Here's the drawing with two shaded views (mm, measured from the low corner). I have some questions. A direction names the side the tool comes from. Round coordinates to 2 decimals unless told otherwise and drop trailing zeros. Loops run counter-clockwise (first coordinate to the right, second up) from the corner with the lowest first, then second, coordinate; pieces in that order, holes last.
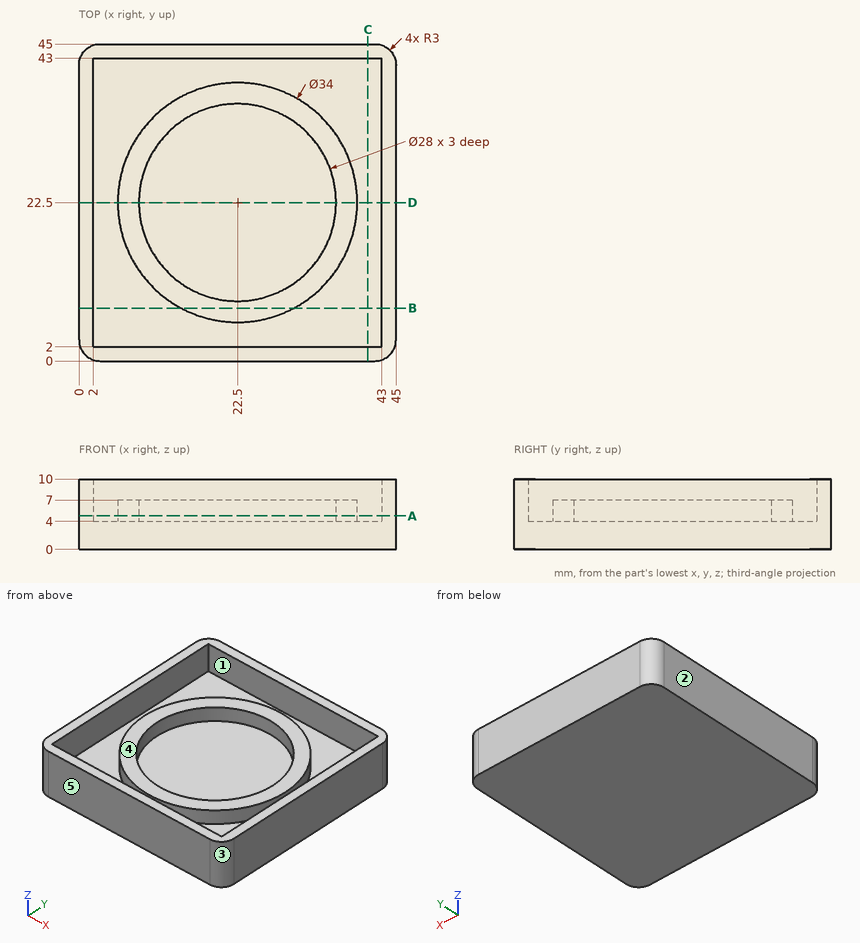
(1) If we section it at C-C, the plane x = 41: List the corners of the cut face in (y, z) for me.
Worked answers:
outline: (0, 0) - (45, 0) - (45, 10) - (43, 10) - (43, 4) - (2, 4) - (2, 10) - (0, 10) - close
(2) If we mould it in two halves opening along X, with no side actions, what happens to the marked faces 3, 4 and 5? For each: released by +X, released by -X, zero draft, split by the parting line, or undercut.
Worked answers:
face 3: released by +X
face 4: undercut
face 5: zero draft
(3) If we section it at A-A, the plane z = 4.75: List the corners of the cut face in (x, y) for me.
Worked answers:
outline: (0, 3) arc R3 ccw to (3, 0) - (42, 0) arc R3 ccw to (45, 3) - (45, 42) arc R3 ccw to (42, 45) - (3, 45) arc R3 ccw to (0, 42) - close; circle Ø34 at (22.5, 22.5); hole (2, 2) - (43, 2) - (43, 43) - (2, 43) - close; hole circle Ø28 at (22.5, 22.5)
(4) If we section it at D-D, the plane y = 22.5: List the corners of the cut face in (x, z) for me, then the cut area to 3 significant figures.
Worked answers:
outline: (0, 0) - (45, 0) - (45, 10) - (43, 10) - (43, 4) - (39.5, 4) - (39.5, 7) - (36.5, 7) - (36.5, 4) - (8.5, 4) - (8.5, 7) - (5.5, 7) - (5.5, 4) - (2, 4) - (2, 10) - (0, 10) - close
area: 222 mm2
(5) Will this pin go through, and if not, where does the flat tip stop? P1, Ø14, axis at x = 25.5, y = 19, coming from the +Z side.
Worked answers:
P1: stops at z = 4
(6) If I drill on line 1 (Y direction, x = 22.5, z = 5.35); line 2 (X direction, y = 3, z = 8.5), over which ranges is the centre line in solid material (lowest first)?
Worked answers:
line 1: y = 0 to 2, 5.5 to 8.5, 36.5 to 39.5, 43 to 45
line 2: x = 0 to 2, 43 to 45
(7) For the marked faces 1 and 2, which set-ups out of +Z, -Z, +X, -X, +Y, -Y let a thin tool reach every point of the face, with its end or its side?
Worked answers:
face 1: +Z
face 2: +Z, -Z, -X, +Y, -Y
(8) If we section it at B-B, the plane y = 7.5: List the corners of the cut face in (x, z) for me.
Worked answers:
outline: (0, 0) - (45, 0) - (45, 10) - (43, 10) - (43, 4) - (30.5, 4) - (30.5, 7) - (14.5, 7) - (14.5, 4) - (2, 4) - (2, 10) - (0, 10) - close
